Geometry: final body of the model. Coordinates: model frame, mm. A direction names the side the tool comes from. Round coordinates to 2 decimals unless told otherwise and drop trailing zeros. Order: outer loops, then holes, each group sorted by start corner. A loop starts at its lowest first (then second) coordinate and runs counter-clockwise, first axis right, second up. Notation, with made-up numbers: M 65,-29.75 L 111,-29.75 A14 cw 111,-24.75 Z; hole C 78,20 d3. An arc over 180 degrees is marked long. Return JSON: item names as keys, results as strings. Group by question number.
Q1. Cut plane A-A on x = -443. Output: boundary loops of the cut face in (y, z).
Q2. Ray query, probe 1 along Y at (x, z) = (449, 26.5); probe 2 along X at (y, z) = (-33.5, -41); probe 3 along X at (y, z) = (-411.5, 96.5). Return the intervals inside material, ascending.
Q3. Cut plane D-D on z = 106.5. Output: boundary loops of the cut face in (x, y).
Q4. Access query for faces 1 (the face through (-8, -600, 57)), 2 (the face through (499, -430, 2)), 3 (the face through (-501, -430, 2)). Directions: +Z, -Z, +X, -X, +Y, -Y. A direction counts if a zero-diameter tool reaches every point of the face in a straight line with its end or side. Return the directions, or none.
Q5. Mould query, pull axis X, two halves, no side actions, for faces 4 (the face through (-400, -302, 2)), 5 (the face through (-501, -170, 2)), 6 (the face through (-3.958, -295.8, 54.956)). Classes: released by +X, released by -X, zero draft, split by the parting line, or undercut.
Q6. Cut plane C-C on y = -256. Output: boundary loops of the cut face in (x, z), and give its area (3 significant figures).
Q7. Cut plane B-B on z = -92. Output: boundary loops of the cut face in (x, y).
Q8. Contact query for flat-ended pins moving along their axis: pin 1 (4 mm diameter, centred on x = 287.5, z = 19, fed in from +Y); pin 2 (3 mm diameter, centred on y = -213, z = -52.5, fed in from +X); pin 3 (1 mm diameter, centred on x = -90, y = -265, fed in from -Z). Output: stop coordinate, or through.
```python
from build123d import *

# Parameters (mm, degrees)
F1_DEPTH = 600
F2_W     = 200
F2_H     = 260
F3_DEPTH = 250.001
F4_W     = 200
F4_H     = 260
F5_DEPTH = 250.001


with BuildPart() as f1:
    # F0 (on Front) → F1 (new body)
    with BuildSketch(Plane.XZ):
        with BuildLine():
            Line((600, 125), (-600, 125))
            Line((-600, 125), (-600, -125))
            Line((-600, -125), (-180, -125))
            ThreePointArc((-180, -125), (0, 55), (180, -125))
            Line((180, -125), (600, -125))
            Line((600, -125), (600, 125))
        make_face()
    extrude(amount=F1_DEPTH)

    # F2 (on face) → F3 (cut, through all)
    with BuildSketch(Plane.XY.offset(125)):
        with Locations((500, -300)):
            Rectangle(F2_W, F2_H)
    extrude(amount=-F3_DEPTH, mode=Mode.SUBTRACT)

    # F4 (on face) → F5 (cut, through all)
    with BuildSketch(Plane.XY.offset(125)):
        with Locations((-500, -300)):
            Rectangle(F4_W, F4_H)
    extrude(amount=-F5_DEPTH, mode=Mode.SUBTRACT)


solid = f1.part
```
Result sheet:
{
 "1": {"outline": "M -600,-125 L -430,-125 L -430,125 L -600,125 Z; M -170,-125 L 0,-125 L 0,125 L -170,125 Z"},
 "2": {"probe 1": "y = -600 to -430, -170 to 0", "probe 2": "x = -600 to -159.2, 159.2 to 600", "probe 3": "x = -400 to 400"},
 "3": {"outline": "M -600,-600 L 600,-600 L 600,-430 L 400,-430 L 400,-170 L 600,-170 L 600,0 L -600,0 L -600,-170 L -400,-170 L -400,-430 L -600,-430 Z"},
 "4": {"face 1": "+Z, -Z, +X, -X, -Y", "face 2": "+Z, -Z, +X", "face 3": "+Z, -Z, -X"},
 "5": {"face 4": "released by -X", "face 5": "zero draft", "face 6": "undercut"},
 "6": {"outline": "M -400,-125 L -180,-125 A180 cw 180,-125 L 400,-125 L 400,125 L -400,125 Z", "area": "149,000 mm²"},
 "7": {"outline": "M -600,-600 L -176.95,-600 L -176.95,0 L -600,0 L -600,-170 L -400,-170 L -400,-430 L -600,-430 Z; M 176.95,-600 L 600,-600 L 600,-430 L 400,-430 L 400,-170 L 600,-170 L 600,0 L 176.95,0 Z"},
 "8": {"pin 1": "stops at y = 0", "pin 2": "stops at x = 400", "pin 3": "stops at z = 30.59"}
}
